```python
from build123d import *

# Parameters (mm, degrees)
BOSS_EXTRUDE1_DEPTH = 4.572
FILLET3_R           = 1.27
FILLET4_R           = 1.27
FILLET5_R           = 1.27
FILLET6_R           = 1.27


with BuildPart() as part:
    # Sketch1 → Boss-Extrude1 (new body)
    with BuildSketch(Plane.XY):
        Polygon((60.901141121, 14.532138101), (60.901141121, -14.423861899), (-0.058858879, -14.423861899), (-61.018858879, -14.423861899), (-61.018858879, 14.532138101), (-0.058858879, 14.532138101), align=None)
        with BuildLine():
            ThreePointArc((-7.625635449, 7.93030318), (-10.980858879, 0.054138101), (-7.625635449, -7.822026977))
            Line((-7.625635449, -7.822026977), (7.507917691, -7.822026977))
            ThreePointArc((7.507917691, -7.822026977), (10.863141121, 0.054138101), (7.507917691, 7.93030318))
            Line((7.507917691, 7.93030318), (-7.625635449, 7.93030318))
        make_face(mode=Mode.SUBTRACT)
    extrude(amount=BOSS_EXTRUDE1_DEPTH)

    # Fillet3
    fillet3_edges = [part.edges().sort_by_distance(p)[0] for p in [
        (-61.018858879, 14.532138101, 2.286),
    ]]
    fillet(fillet3_edges, radius=FILLET3_R)

    # Fillet4
    fillet4_edges = [part.edges().sort_by_distance(p)[0] for p in [
        (-61.018858879, -14.423861899, 2.286),
    ]]
    fillet(fillet4_edges, radius=FILLET4_R)

    # Fillet5
    fillet5_edges = [part.edges().sort_by_distance(p)[0] for p in [
        (60.901141121, -14.423861899, 2.286),
    ]]
    fillet(fillet5_edges, radius=FILLET5_R)

    # Fillet6
    fillet6_edges = [part.edges().sort_by_distance(p)[0] for p in [
        (60.901141121, 14.532138101, 2.286),
    ]]
    fillet(fillet6_edges, radius=FILLET6_R)


solid = part.part
```
Source: CAD feature listing. Evaluate the final solid. Frame: model axes, mm. A direction names the side the tool comes from. Give positions to 0.01 mm unless a question says otherwise; leave off trailing zeros. Loops run counter-clockwise (first coordinate to the right, second up) from the corner with the lowest first, then second, coordinate; pieces in that order, holes last. Notation, with made-up numbers: (81.25, 31) - (123.25, 31) arc R23 cw to (123.25, 63) - close; hole circle Ø10 at (49.5, 80). An arc over 180 degrees is marked (long way). Use CSV: the item, a comma, the result in double quotes.
1) Line query: line 1 (Y direction, x = -5, z = 1.4); line 2 (X direction, y = 2.75, z = 0.7); line 3 (X direction, y = 4.25, z = 3.6). Output: solid intervals per line, ascending.
Worked out:
line 1,"y = -14.42 to -7.82, 7.93 to 14.53"
line 2,"x = -61.02 to -10.64, 10.53 to 60.9"
line 3,"x = -61.02 to -10.14, 10.03 to 60.9"
2) Cut plane C-C (y = -6.25). Output: boundary loops of the cut face in (x, z), and give its area (3 significant figures).
Worked out:
outline,"(-61.02, 0) - (-8.98, 0) - (-8.98, 4.57) - (-61.02, 4.57) - close; (8.86, 0) - (60.9, 0) - (60.9, 4.57) - (8.86, 4.57) - close"
area,"476 mm^2"
3) Set-up query: faces 5 (the flat face through (-61.019, 0, 2)), 6 (the cylindrical face through (10.862, -0.069, 2.254)). Return all of +Z, -Z, +X, -X, +Y, -Y with unobstructed straight access to the full face (end or side cutting, diameter ignored); none if empty.
Worked out:
face 5,"+Z, -Z, -X, +Y, -Y"
face 6,"+Z, -Z"
4) Cut plane A-A (z = 3.65). Output: boundary loops of the cut face in (x, y).
Worked out:
outline,"(-61.02, -13.15) arc R1.27 ccw to (-59.75, -14.42) - (59.63, -14.42) arc R1.27 ccw to (60.9, -13.15) - (60.9, 13.26) arc R1.27 ccw to (59.63, 14.53) - (-59.75, 14.53) arc R1.27 ccw to (-61.02, 13.26) - close; hole (-7.63, -7.82) - (7.51, -7.82) arc R10.92 ccw to (7.51, 7.93) - (-7.63, 7.93) arc R10.92 ccw to start"
5) Cut plane B-B (y = 3.25). Output: boundary loops of the cut face in (x, z).
Worked out:
outline,"(-61.02, 0) - (-10.5, 0) - (-10.5, 4.57) - (-61.02, 4.57) - close; (10.39, 0) - (60.9, 0) - (60.9, 4.57) - (10.39, 4.57) - close"
6) Mould query, pull axis Y, two halves, no side actions, for faces 1 (the flat face through (0, 7.93, 2)), 2 (the flat face through (1, 10, 4.572)), 3 (the flat face through (1, 14.532, 2)), 4 (the flat face through (-1, -14.424, 2)). Classes: +Y half, -Y half, draft (parallel to the pull), parting line (faces both ways), or undercut.
Worked out:
face 1,"undercut"
face 2,"draft"
face 3,"+Y half"
face 4,"-Y half"
